Autodesk Fusion 360 part; units mm, degrees
sketch "Sketch1" plane through (0, 0, 0) normal (0, 1, 0) x (1, 0, 0)
  line L0 (0, 0) -> (78, 0)
  line L1 (0, 0) -> (0, -8)
  line L2 (0, -8) -> (24, -8)
  line L3 (24, -8) -> (47.3154, -58)
  line L4 (47.3154, -58) -> (62.8659, -50.7487)
  line L5 (47.6516, -18.1216) -> (52.1832, -16.0085)
  line L6 (52.1832, -16.0085) -> (67.3974, -48.6356)
  line L7 (78, 0) -> (78, -43.6915)
  line L8 (67.3974, -48.6356) -> (78, -43.6915)
  line L9 (0, -8) -> (0, -16)
  line L10 (0, -16) -> (24, -16)
  line L11 (24, -16) -> (24, -34)
  line L12 (47.6516, -18.1216) -> (62.8659, -50.7487)
  line L13 (24, -34) -> (36.124, -34)
  dimension "d1" = 78
  dimension "d2" = 8
  dimension "d3" = 24
  dimension "d4" = 8
  dimension "d5" = 24
  dimension "d6" = 18
  dimension "d7" = 65
  dimension "d8" = 36
  dimension "d9" = 50
  dimension "d10" = 36
  dimension "d11" = 36
  dimension "d12" = 5
  dimension "d13" = 17.1581
extrude "Extrude1" add sketch "Sketch1" along normal blind 28
sketch "Sketch2" plane through (0, 0, 0) normal (0, -1, 0) x (1, 0, 0)
  line L0 (0, 16) -> (0, 0)
  line L1 (0, 0) -> (78, 0)
  line L2 (78, 0) -> (78, 43.6915)
  line L3 (78, 43.6915) -> (67.3974, 48.6356)
  line L4 (67.3974, 48.6356) -> (52.1832, 16.0085)
  line L5 (52.1832, 16.0085) -> (47.6516, 18.1216)
  line L6 (47.6516, 18.1216) -> (62.8659, 50.7487)
  line L7 (62.8659, 50.7487) -> (47.3154, 58)
  line L8 (47.3154, 58) -> (36.124, 34)
  line L9 (36.124, 34) -> (24, 34)
  line L10 (24, 34) -> (24, 16)
  line L11 (24, 16) -> (0, 16)
  line L12 (0, 0) -> (24, 0) construction
  line L13 (24, 0) -> (24, 8) construction
  line L14 (24, 16) -> (0, 16) construction
  line L15 (0, 16) -> (0, 0) construction
  line L16 (24, 0) -> (0, 0) construction
  line L17 (0, 0) -> (0, 8) construction
  line L18 (0, 8) -> (24, 8) construction
  line L19 (24, 8) -> (24, 0) construction
  line L20 (24, 16) -> (24, 34) construction
  line L21 (24, 34) -> (36.124, 34) construction
  line L22 (36.124, 34) -> (24, 8) construction
  line L23 (0, 8) -> (0, 16)
  line L24 (0, 16) -> (24, 16)
  line L25 (24, 16) -> (24, 34)
  line L26 (24, 34) -> (36.124, 34)
  line L27 (36.124, 34) -> (24, 8)
  line L28 (24, 8) -> (0, 8)
  dimension "d16" = 8
extrude "Extrude2" cut sketch "Sketch2" against normal blind 10 contours L0 L9 L10 L11 L23 L24 L25 L26 L27 L28
sketch "Sketch3" plane through (30.6661, 0, 65.7637) normal (0.4226, 0, 0.9063) x (0, 1, 0)
  line L0 (0, -18.3704) -> (0, -35.5285)
  line L1 (0, -35.5285) -> (28, -35.5285)
  line L2 (28, -35.5285) -> (28, -18.3704)
  line L3 (28, -18.3704) -> (0, -18.3704)
  line L4 (0, -18.3704) -> (28, -18.3704) construction
  line L5 (28, -18.3704) -> (28, -35.5285) construction
  line L6 (28, -35.5285) -> (0, -35.5285) construction
  line L7 (0, -35.5285) -> (0, -18.3704) construction
  line L8 (0, -35.5285) -> (28, -35.5285) construction
  line L9 (28, -35.5285) -> (28, -26.9495) construction
  line L10 (28, -26.9495) -> (0, -26.9495) construction
  line L11 (0, -26.9495) -> (0, -35.5285) construction
  line L12 (0, -26.9495) -> (28, -26.9495) construction
  line L13 (28, -26.9495) -> (28, -34.4495) construction
  line L14 (28, -34.4495) -> (0, -34.4495) construction
  line L15 (0, -34.4495) -> (0, -26.9495) construction
  line L16 (0, -26.9495) -> (28, -26.9495) construction
  line L17 (28, -26.9495) -> (28, -19.4495) construction
  line L18 (28, -19.4495) -> (0, -19.4495) construction
  line L19 (0, -19.4495) -> (0, -26.9495) construction
  line L20 (0, -35.5285) -> (7, -35.5285) construction
  line L21 (7, -35.5285) -> (7, -18.3704) construction
  line L22 (7, -18.3704) -> (0, -18.3704) construction
  line L23 (0, -18.3704) -> (0, -35.5285) construction
  line L24 (28, -35.5285) -> (21, -35.5285) construction
  line L25 (21, -35.5285) -> (21, -18.3704) construction
  line L26 (21, -18.3704) -> (28, -18.3704) construction
  line L27 (28, -18.3704) -> (28, -35.5285) construction
  circle A0 centre (7, -26.9495) radius 3
  circle A1 centre (21, -26.9495) radius 3
  dimension "d19" = 28
  dimension "d20" = 7.5
  dimension "d21" = 28
  dimension "d22" = 7.5
  dimension "d23" = 7
  dimension "d24" = 7
  dimension "d25" = 6
  dimension "d26" = 6
extrude "Extrude3" add sketch "Sketch3" along normal blind 6 contours A0 | A1
Geometry check sheet. Reference: the model listing, model coordinates, mm. A direction names the side the tool comes from. Give positions to 0.01 mm unless a question says otherwise; leave off trailing zeros. Write each loop counter-clockwise with the first axis right and the second up, starting at its lowest first coordinate (ties: lowest second). Pieces come first, ordered by that corner, then holes. Notation, with made-up numbers: (57, 83.25) -> (73, 83.25) arc R17 cw to (73, 115.25) -> close; hole circle Ø3 at (50.25, -20). An arc over 180 degrees is marked (long way). Use one line per item in the form item = value.
Item 1: Depth check by flat-ended pin: pin 1 Ø2 at (x, y) = (62, 15) entering from +Z; pin 2 Ø12 at (x, z) = (22.5, 27.5) entering from -Y; pin 3 Ø5.5 at (x, y) = (12, 16) entering from +Z. Enter the tip coordinate at first touch or a pass-through.
Results list:
pin_1 = 51.62
pin_2 = 10
pin_3 = 16
Item 2: Sectioned sample at B-B on y = 13. Enter the section's corners in (x, z).
Results list:
outline = (0, 0) -> (78, 0) -> (78, 43.69) -> (67.4, 48.64) -> (52.18, 16.01) -> (47.65, 18.12) -> (62.87, 50.75) -> (47.32, 58) -> (36.12, 34) -> (24, 34) -> (24, 16) -> (0, 16) -> close
Item 3: Sectioned sample at A-A on z = 45.5. Enter the section's corners in (x, y).
Results list:
outline = (41.49, 0) -> (60.42, 0) -> (60.42, 28) -> (41.49, 28) -> close; (65.94, 0) -> (74.12, 0) -> (74.12, 28) -> (65.94, 28) -> close
Item 4: Sectioned sample at C-C on x = 6.5. Enter the section's corners in (y, z), plus the area to 3 significant figures.
Results list:
outline = (0, 0) -> (28, 0) -> (28, 16) -> (10, 16) -> (10, 8) -> (0, 8) -> close
area = 368 mm2
Item 5: Mould release check, pull along Z, two halves, no side actions. Record for faces 6 (the flat face through (38, 14, 0)), 7 (the flat face through (59.68, 13.8, 32.09)), 8 (the flat face through (72.62, 13.8, 46.2)), 9 (the flat face through (18, 10, 15)): released by +Z, released by -Z, zero draft, split by the parting line, or undercut.
Results list:
face_6 = released by -Z
face_7 = undercut
face_8 = released by +Z
face_9 = zero draft
Item 6: Scan lines: line 1 (Z direction, x = 58.5, y = 8.25); line 2 (X direction, y = 24, z = 27); line 3 (X direction, y = 13, z = 40). Record each from-to range of solid material in increasing order.
Results list:
line_1 = 0 to 29.55, 41.39 to 52.78, 55.23 to 59.4
line_2 = 24 to 51.79, 57.31 to 78
line_3 = 38.92 to 57.85, 63.37 to 78
Item 7: Sectioned sample at D-D on z = 31. Enter the section's corners in (x, y).
Results list:
outline = (24, 10) -> (34.73, 10) -> (34.73, 0) -> (53.66, 0) -> (53.66, 28) -> (24, 28) -> close; (59.17, 0) -> (78, 0) -> (78, 28) -> (59.17, 28) -> close
Item 8: Access from +Z, -Z, +X, -X, +Y, -Y to the whole of each face (thin tool, end or side, straight path). Record for faces 1 (the cylindrical face through (57.16, 23.86, 56.67)), 2 (the flat face through (12, 19, 16)), 3 (the flat face through (47, 28, 22)), 4 (the flat face through (49.89, 13.8, 17.08)), 5 (the flat face through (12, 5, 8)).
Results list:
face_1 = none
face_2 = +Z, -X, +Y, -Y
face_3 = +Z, -Z, +X, -X, +Y
face_4 = +Y, -Y
face_5 = +Z, -X, -Y
